Solid Edge part; units mm, degrees
sketch "Sketch1" plane through (0, 0, 0) normal (0, 0, 1) x (1, 0, 0)
  line L0 (-4.5, -4.5) -> (4.5, -4.5)
  line L1 (4.5, -4.5) -> (4.5, 4.5)
  line L2 (4.5, 4.5) -> (-4.5, 4.5)
  line L3 (-4.5, 4.5) -> (-4.5, -4.5)
extrude "Protrusion1" add sketch "Sketch1" against normal blind 2
sketch "Sketch2" plane through (0, 0, -2) normal (0, 0, -1) x (1, 0, 0)
  line L0 (3.35, 3.35) -> (-3.35, 3.35)
  line L1 (-3.35, 3.35) -> (-3.35, -3.35)
  line L2 (-3.35, -3.35) -> (3.35, -3.35)
  line L3 (3.35, -3.35) -> (3.35, 3.35)
extrude "ExtrudedProtrusion_2" add sketch "Sketch2" along normal blind 2
sketch "Sketch3" plane through (3.35, 0, -3.5) normal (1, 0, 0) x (0, 1, 0)
  line L0 (1.65, -0.5) -> (1.65, 1)
  line L1 (1.65, 1) -> (-1.65, 1)
  line L2 (-1.65, 1) -> (-1.65, -0.5)
  line L3 (-1.65, -0.5) -> (-3.35, -0.5)
  line L4 (-3.35, -0.5) -> (-3.35, 1.5)
  line L5 (-3.35, 1.5) -> (3.35, 1.5)
  line L6 (3.35, 1.5) -> (3.35, -0.5)
  line L7 (3.35, -0.5) -> (1.65, -0.5)
extrude "Protrusion2" add sketch "Sketch3" along normal up to surface (1.15 mm away)
sketch "Sketch4" plane through (0, 0, 0) normal (0, 0, 1) x (0, 1, 0)
  circle A0 centre (0, 0) radius 2
extrude "ExtrudedProtrusion_4" add sketch "Sketch4" along normal blind 1
sketch "Sketch5" plane through (0, 0, 0) normal (0, 0, 1) x (0, 1, 0)
  line L0 (3.25, -1.9691) -> (3.25, -4.5)
  line L1 (3.25, -4.5) -> (3.95, -4.5)
  line L2 (3.95, -4.5) -> (3.95, -2.1558)
  line L3 (-3.95, -4.5) -> (-3.95, -2.1558)
  line L4 (-3.25, -4.5) -> (-3.95, -4.5)
  line L5 (-3.25, -1.9691) -> (-3.25, -4.5)
  arc A0 (-3.25, -1.9691) -> (3.25, -1.9691) centre (0, 0) cw
  arc A1 (-3.95, -2.1558) -> (3.95, -2.1558) centre (0, 0) cw
extrude "Protrusion3" add sketch "Sketch5" along normal blind 10
sketch "Sketch6" plane through (4.5, 0, 0.5) normal (1, 0, 0) x (0, 1, 0)
  line L0 (4.5, -6.5) -> (-4.5, -6.5)
  line L1 (-4.5, -6.5) -> (-4.5, -0.5)
  line L2 (-4.5, -0.5) -> (-3.95, -0.5)
  line L3 (-3.95, -0.5) -> (-3.95, 9.5)
  line L4 (-3.95, 9.5) -> (-3.25, 9.5)
  line L5 (-3.25, 9.5) -> (-3.25, -0.5)
  line L6 (-3.25, -0.5) -> (3.25, -0.5)
  line L7 (3.25, -0.5) -> (3.25, 9.5)
  line L8 (3.25, 9.5) -> (3.95, 9.5)
  line L9 (3.95, 9.5) -> (3.95, -0.5)
  line L10 (3.95, -0.5) -> (4.5, -0.5)
  line L11 (4.5, -0.5) -> (4.5, -6.5)
extrude "ExtrudedProtrusion_8" add sketch "Sketch6" along normal blind 12
sketch "Sketch7" plane through (6.25, 0, 0) normal (0, 0, 1) x (1, 0, 0)
  line L0 (-1.75, -3.25) -> (-1.75, 3.25)
  line L1 (-1.75, 3.25) -> (10.25, 3.25)
  line L2 (10.25, 3.25) -> (10.25, -3.25)
  line L3 (10.25, -3.25) -> (-1.75, -3.25)
extrude "ExtrudedProtrusion_9" add sketch "Sketch7" along normal blind 2
sketch "Sketch8" plane through (0.25, 0, 0) normal (0, 0, 1) x (0, 1, 0)
  line L0 (1.8413, -0.5307) -> (3.45, -2.1393)
  line L1 (3.45, -2.1393) -> (3.45, -4.2607)
  line L2 (0.7807, -1.5913) -> (3.45, -4.2607)
  line L3 (1.8413, -0.5307) -> (0.7807, -1.5913)
  line L4 (1.8413, 1.0307) -> (3.2173, 2.4067)
  line L5 (2.1567, 3.4673) -> (3.2173, 2.4067)
  line L6 (0.7807, 2.0913) -> (2.1567, 3.4673)
  line L7 (0.7807, 2.0913) -> (1.8413, 1.0307)
extrude "ExtrudedProtrusion_6" add sketch "Sketch8" along normal blind 0.5
mirror "Mirror1" about plane through (0.25, 0, 0) normal (0, 1, 0) of "ExtrudedProtrusion_6"
fillet "Round_1" radius 2 1 edges at (4.5, 0, 0)
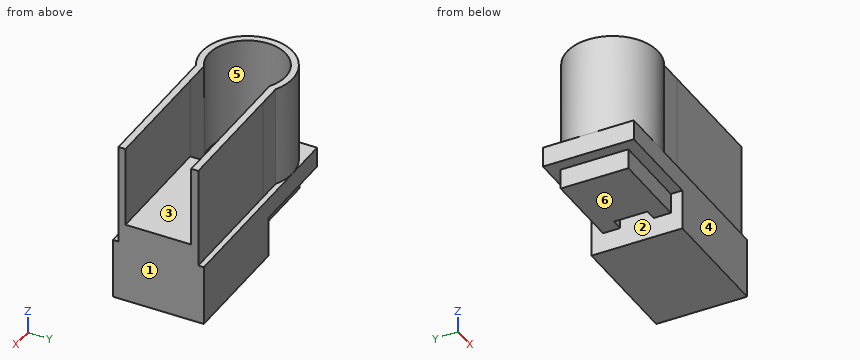
Model file for the job. Use its own axes, mm. Face numbers are marked on the shaded views. A direction names the side the tool comes from. Give positions to 0.01 mm unless a question says otherwise; leave off trailing zeros. Loops run counter-clockwise (first coordinate to the right, second up) from the corner with the lowest first, then second, coordinate; pieces in that order, holes last. Notation, with made-up numbers: (59, 14.5) - (79, 14.5) arc R34 cw to (79, 50.5) - close; hole circle Ø3 at (49, -39.75). An arc over 180 degrees is marked (long way). Use one line per item in the form item = value.
(1) Pull direction X, two halves, no side cores. Call the marked faces 1, 2 and 3: pulls with the +X half, pulls with the -X half, needs draft (parallel to the pull), parting line crosses it, or undercut.
Determined:
face_1 = pulls with the +X half
face_2 = undercut
face_3 = needs draft
(2) Cut at A-A (z = 9.25). Give the cut face in (x, y), then the cut area to 3 significant figures.
Determined:
outline = (1.97, -3.25) arc R3.8 cw (long way) to (1.97, 3.25) - (4.5, 3.25) - (16.5, 3.25) - (16.5, 3.95) - (4.5, 3.95) - (2.16, 3.95) arc R4.5 ccw (long way) to (2.16, -3.95) - (4.5, -3.95) - (16.5, -3.95) - (16.5, -3.25) - (4.5, -3.25) - close
area = 32.4 mm^2
(3) 3-axis set-ups, long thin cutter, end or side, ignore diameter. For the marked faces 4, 5 and 6: which of +Z, -Z, +X, -X, +Y, -Y reach the whole face in a straight line?
Determined:
face_4 = +Z, -Z, +X, -X, -Y
face_5 = +Z
face_6 = -Z, -X, +Y, -Y
(4) Drop flat-ended pins along their axis: P1, Ø0.6, axis at x = 3.5, y = 0, coming from the -Z side; P2, Ø3, axis at x = 8, z = 5.5, coming from the +Y side; P3, Ø2, axis at y = 2, z = 4, coming from the -X side. Give the stop position or say it passes through.
Determined:
P1 = -4
P2 = 3.95
P3 = -4.39
(5) Cut at B-B (x = 12.75). Give the cut face in (y, z), then the cut area to 3 significant figures.
Determined:
outline = (-4.5, -6) - (4.5, -6) - (4.5, 0) - (3.95, 0) - (3.95, 10) - (3.25, 10) - (3.25, 2) - (-3.25, 2) - (-3.25, 10) - (-3.95, 10) - (-3.95, 0) - (-4.5, 0) - close
area = 81.0 mm^2
(6) Drill centre lines: L1, parallel to Y at x = 0, z = 2; L2, parallel to Y at x = 2.25, z = 6.5; L3, parallel to X at y = 0, z = -3.25. Where is each one in solid material? Low to high.
Determined:
L1 = -4.5 to -3.8, 3.8 to 4.5
L2 = -3.95 to -3.25, 3.25 to 3.95
L3 = -3.35 to 3.35, 4.5 to 16.5
